Autodesk Inventor part; units mm, degrees
ref_plane "YZ Plane" through (0, 0, 0) normal (1, 0, 0) x (0, 1, 0)
ref_plane "XZ Plane" through (0, 0, 0) normal (0, 1, 0) x (-1, 0, 0)
ref_plane "XY Plane" through (0, 0, 0) normal (0, 0, 1) x (1, 0, 0)
sketch "Szkic1" plane through (0, 0, 0) normal (0, 0, 1) x (1, 0, 0)
  line L0 (206.45, -143.65) -> (206.45, -129.275)
  line L1 (206.45, -129.275) -> (220.2, -129.275)
  line L2 (206.45, -143.65) -> (220.2, -143.65)
  line L3 (220.2, -129.275) -> (220.2, -143.65)
extrude "Wyciągnięcie proste1" add sketch "Szkic1" against normal blind 5.2
fillet "Zaokrąglenie1" radius 0.5 1 edges at (220.2, -136.4625, -5.2)
sketch "Szkic6" plane through (0, 0, 0) normal (0, 0, 1) x (1, 0, 0)
  arc A0 (213.325, -135.3377) -> (213.325, -137.5873) centre (213.325, -136.4625) ccw
  circle A1 centre (213.325, -136.4625) radius 1.3125
  line L0 (213.4625, -134.4622) -> (213.1875, -134.4622)
  line L1 (213.1875, -134.4622) -> (213.1875, -134.9872)
  line L2 (213.1875, -134.9872) -> (213.4625, -134.9872)
  line L3 (213.4625, -134.9872) -> (213.4625, -134.4622)
  line L4 (210.4962, -136.4625) -> (213.325, -133.6337) construction
  line L5 (212.0078, -134.9509) -> (211.8134, -135.1453)
  line L6 (211.8134, -135.1453) -> (212.1846, -135.5166)
  line L7 (212.1846, -135.5166) -> (212.3791, -135.3221)
  line L8 (212.3791, -135.3221) -> (212.0078, -134.9509)
  line L9 (211.3247, -138.4628) -> (211.3247, -134.4622) construction
  line L10 (211.3247, -136.325) -> (211.3247, -136.6)
  line L11 (211.3247, -136.6) -> (211.8497, -136.6)
  line L12 (211.8497, -136.6) -> (211.8497, -136.325)
  line L13 (211.8497, -136.325) -> (211.3247, -136.325)
  line L14 (213.325, -139.2913) -> (210.4962, -136.4625) construction
  line L15 (211.8134, -137.7797) -> (212.0078, -137.9741)
  line L16 (212.0078, -137.9741) -> (212.3791, -137.6029)
  line L17 (212.3791, -137.6029) -> (212.1846, -137.4084)
  line L18 (212.1846, -137.4084) -> (211.8134, -137.7797)
  line L19 (215.3253, -138.4628) -> (211.3247, -138.4628) construction
  line L20 (213.1875, -138.4628) -> (213.4625, -138.4628)
  line L21 (213.4625, -138.4628) -> (213.4625, -137.9378)
  line L22 (213.4625, -137.9378) -> (213.1875, -137.9378)
  line L23 (213.1875, -137.9378) -> (213.1875, -138.4628)
  line L24 (216.1538, -136.4625) -> (213.325, -139.2913) construction
  line L25 (214.6422, -137.9741) -> (214.8366, -137.7797)
  line L26 (214.8366, -137.7797) -> (214.4654, -137.4084)
  line L27 (214.4654, -137.4084) -> (214.2709, -137.6029)
  line L28 (214.2709, -137.6029) -> (214.6422, -137.9741)
  line L29 (215.3253, -134.4622) -> (215.3253, -138.4628) construction
  line L30 (215.3253, -136.6) -> (215.3253, -136.325)
  line L31 (215.3253, -136.325) -> (214.8003, -136.325)
  line L32 (214.8003, -136.325) -> (214.8003, -136.6)
  line L33 (214.8003, -136.6) -> (215.3253, -136.6)
  line L34 (213.325, -133.6337) -> (216.1538, -136.4625) construction
  line L35 (214.8366, -135.1453) -> (214.6422, -134.9509)
  line L36 (214.6422, -134.9509) -> (214.2709, -135.3221)
  line L37 (214.2709, -135.3221) -> (214.4654, -135.5166)
  line L38 (214.4654, -135.5166) -> (214.8366, -135.1453)
  line L39 (213.325, -136.4625) -> (213.325, -135.3377)
  line L40 (213.325, -136.4625) -> (213.325, -137.5873)
  point P0 (211.3247, -134.4622)
  point P1 (213.325, -134.7247)
  point P2 (212.0962, -135.2337)
  point P3 (211.5872, -136.4625)
  point P4 (212.0962, -137.6913)
  point P5 (213.325, -138.2003)
  point P6 (214.5538, -137.6913)
  point P7 (215.0628, -136.4625)
  point P8 (214.5538, -135.2337)
  dimension "d55" = 2.625
  dimension "d57" = 0.275
  dimension "d61" = 360
fillet "Zaokrąglenie2" radius 1 1 edges at (220.2, -136.4625, 0)
extrude "Wyciągnięcie proste5" add sketch "Szkic6" along normal blind 0.001 contours L39 L40 A0 | A1 | L3 L2 L1 L0 | L8 L7 L6 L5 | L13 L12 L11 L10 | L18 L17 L16 L15 | L23 L22 L21 L20 | L28 L27 L26 L25 | L33 L32 L31 L30 | L38 L37 L36 L35
properties part number "PRZYCISK IO" material "Tworzywo sztuczne, nieprzezroczyste czarne"
The model under review builds one solid part; all positions refer to its coordinate system, in mm. Give positions to 0.01 mm unless a question says otherwise; leave off trailing zeros. Write each question's results on one line, items separated by ' | '.
1) Insertion check: pin 1 Ø1 at (x, y) = (208, -131) entering from +Z. The pin has a flat end and moves straight along its axis. Give the tip position at first contact, or say it passes through.
Conclusion:
pin 1: stops at z = 0
2) Draft analysis for pull direction Y (two halves, no side actions). For faces 1 (the face through (213, -143.65, -3)), 2 (the face through (219.915, -136.563, -0.301)), 3 (the face through (213, -129.275, -3)), state which applies: pulls with the +Y half, pulls with the -Y half, needs draft (parallel to the pull), parting line crosses it, or undercut.
Conclusion:
face 1: pulls with the -Y half | face 2: needs draft | face 3: pulls with the +Y half
3) For line 1 along Z through (x, y) = (211.75, -132); line 2 along X through (y, z) = (-131.75, -0.15); line 3 along X through (y, z) = (-134.5, -0.65), list the stretches that pass through material, from the lowest coordinate up. Write a range as from..to.
Conclusion:
line 1: z = -5.2..0 | line 2: x = 206.45..219.73 | line 3: x = 206.45..220.14
